The drawing under review shows one solid part. Ordinate dimensions are in mm from its lowest x, y, z. A direction names the side the tool comes from. Give positions to 0.01 mm unless a question says otherwise; leave off trailing zeros. Write each loop counter-clockwise with the first axis right and the second up, starting at its lowest first coordinate (ties: lowest second). Pieces come first, ordered by that corner, then holes.
Q1. We need section C-C (x = 30). Write out the cut boundary in (y, z), then the cut area to 3 significant figures.
Q2. We need section D-D (x = 24.5). Write out the cut boundary in (y, z), then the cut area to 3 significant figures.
Q3. Insertion check: P1, Ø5, axis at x = 30, y = 9, coming from the +Z side; P2, Ø2, axis at x = 28.5, z = 3.5, coming from the -Y side; P3, Ø0.6, axis at y = 6.5, z = 5.5, coming from the -X side. Each pin has a flat end and moves straight along its axis. Give the tip position at first contact, or say it passes through.
Q4. For line 1 (X direction, y = 11, z = 5.05); line 2 (Z direction, x = 28.5, y = 2); line 3 (X direction, y = 8.5, z = 4.05) (1 decimal), list the stretches that pass through material, from the lowest coordinate up.
Q5. Machinability: for the marked faces 1, 2 and 3, which of the approach directions +Z, -Z, +X, -X, +Y, -Y give a long, thin tool a straight path to every point of the face, cutting with its end or side? Answer none if there is none.
Q6. We need section A-A (z = 3.8). Write out the cut boundary in (x, y) (1 decimal).
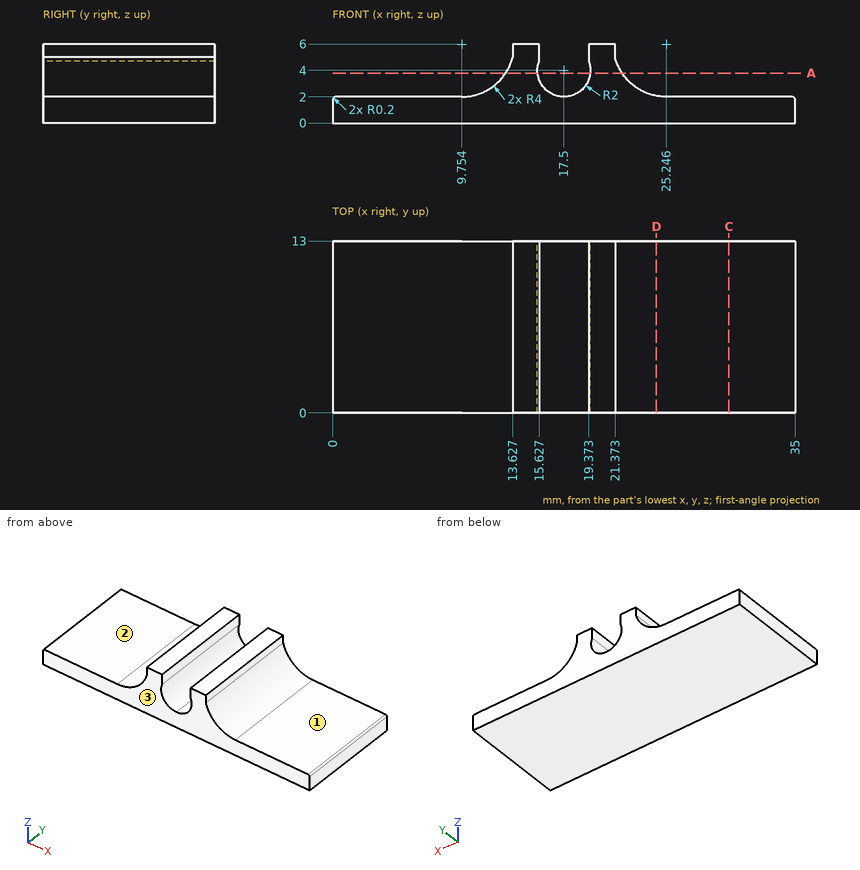
Computed:
1. outline: (0, 0) - (13, 0) - (13, 2) - (0, 2) - close
1. area: 26.0 mm2
2. outline: (0, 0) - (13, 0) - (13, 2.07) - (0, 2.07) - close
2. area: 26.9 mm2
3. P1: stops at z = 2
3. P2: passes through
3. P3: stops at x = 13.63
4. line 1: x = 13.63 to 15.63, 19.37 to 21.37
4. line 2: z = 0 to 2
4. line 3: x = 13.2 to 15.5, 19.5 to 21.8
5. face 1: +Z, +X, +Y, -Y
5. face 2: +Z, -X, +Y, -Y
5. face 3: +Z, -Z, +X, -X, -Y
6. outline: (13.1, 0) - (15.5, 0) - (15.5, 13) - (13.1, 13) - close; (19.5, 0) - (21.9, 0) - (21.9, 13) - (19.5, 13) - close
